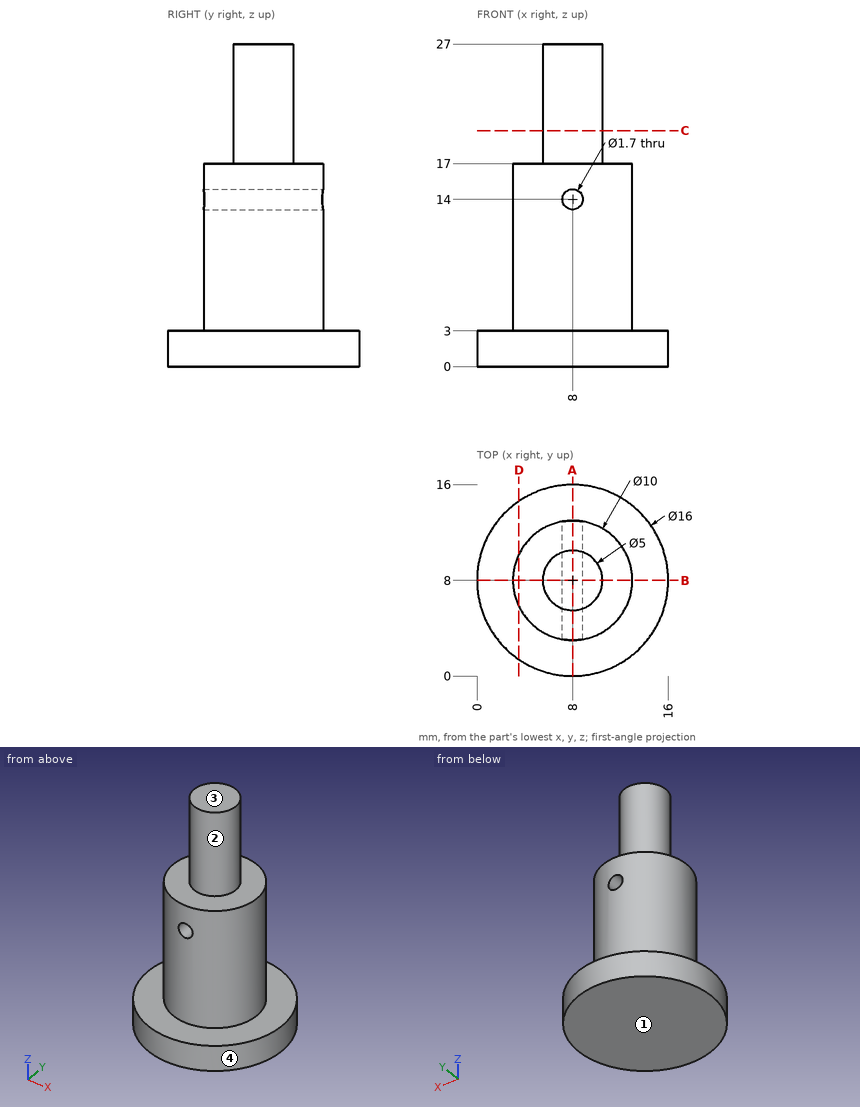
Geometry check sheet. Reference: drawing and pictorial views, mm from the part's lowest x, y, z. A direction names the side the tool comes from. Round coordinates to 2 decimals unless told otherwise and drop trailing zeros. Order: outer loops, then holes, each group sorted by start corner. A loop starts at its lowest first (then second) coordinate and runs counter-clockwise, first axis right, second up. Notation, with made-up numbers: M 35,35 L 62,35 A27 ccw 62,63 Z; hole C 1,11.25 d11. An arc over 180 degrees is marked long. One line per item, written item: value. Start each with the question number.
1. Section check D-D on x = 3.5. Enter the section's corners in (y, z), and give its area (3 significant figures).
2. Section check A-A on x = 8. Enter the section's corners in (y, z), and give its area (3 significant figures).
3. Scan lines: line 1 along Z through (x, y) = (8, 8.75); line 2 along Z through (x, y) = (8, 11.25); line 3 along Z through (x, y) = (3.75, 14.5). Record each from-to range of solid material in increasing order.
4. Section check C-C on z = 19.75. Enter the section's corners in (x, y), and give its area (3 significant figures).
5. Access from +Z, -Z, +X, -X, +Y, -Y to the whole of each face (thin tool, end or side, straight path). Record for the marked faces 1 and 2.
6. Release check for a two-part mould opening along X. For the marked faces 3 and 4 record: released by +X, released by -X, zero draft, split by the parting line, or undercut.
7. Gauge pin test, flat ends, axial feed: P1, Ø8, axis at x = 5, z = 13, coming from the -Y side; P2, Ø1.4, axis at x = 8, z = 14, coming from the -Y side (3 decimals); P3, Ø6, axis at y = 8.5, z = 7.5, coming from the -X side; P4, Ø3, axis at x = 3, y = 4.5, coming from the +Z side. Record the tip position at first contact, or that the pin passes through.
8. Section check B-B on y = 8. Enter the section's corners in (x, z).
Results found:
1. outline: M 1.39,0 L 14.61,0 L 14.61,3 L 10.18,3 L 10.18,17 L 5.82,17 L 5.82,3 L 1.39,3 Z
1. area: 101 mm^2
2. outline: M 0,0 L 16,0 L 16,3 L 13,3 L 13,13.15 L 3,13.15 L 3,3 L 0,3 Z; M 3,14.85 L 13,14.85 L 13,17 L 10.5,17 L 10.5,27 L 5.5,27 L 5.5,17 L 3,17 Z
2. area: 221 mm^2
3. line 1: 0 to 13.15, 14.85 to 27
3. line 2: 0 to 13.15, 14.85 to 17
3. line 3: 0 to 3
4. outline: C 8,8 d5
4. area: 19.6 mm^2
5. face 1: -Z, +X, -X, +Y, -Y
5. face 2: +Z
6. face 3: zero draft
6. face 4: split by the parting line
7. P1: y = 3
7. P2: through
7. P3: x = 3
7. P4: z = 17
8. outline: M 0,0 L 16,0 L 16,3 L 13,3 L 13,17 L 10.5,17 L 10.5,27 L 5.5,27 L 5.5,17 L 3,17 L 3,3 L 0,3 Z; hole C 8,14 d1.7
